Model file for the job. Use its own axes, mm. A direction names the side the tool comes from. Round coordinates to 2 decimals unless told otherwise and drop trailing zeros. Order: outer loops, then holes, each group sorted by start corner. A loop starts at its lowest first (then second) coordinate and runs counter-clockwise, first axis right, second up. Notation, with made-up numbers: (68.5, 23) - (76.5, 23) arc R20 ccw to (76.5, 52) - close; hole circle Ø6 at (1.25, 70). An arc over 180 degrees is marked (long way). Put each result on its own line as item: value. Start each with the question number.
Item 1: Saw through at A-A on y = 23.9. List the corners of the cut face in (x, z).
Item 2: Which spindle directions (+Z, -Z, +X, -X, +Y, -Y) get a long thin tool onto all of the face, cutting with end or side? Do faces 1 (the face through (-20.5, 31, -12)), 2 (the face through (-24, 7.8, -1)), 3 (the face through (24.86, 32.1, -0.57)). Say none if no direction does.
Item 3: Saw through at C-C on x = -24.2. List the corners of the cut face in (y, z).
Item 4: Pin check, flat tips, straight feed: pin 1 Ø2.5 at (x, z) = (26.5, -17) entering from -Y; pin 2 Ø1.3 at (x, z) = (-19.5, -1.5) entering from +Y; pin 3 Ø4.5 at (x, z) = (-10.6, -9) entering from +Y. Stop position of each tip, or through.
Item 5: Probe probe 1 along X at (y, z) = (32, -19.1); probe 2 along Z at (x, y) = (-24, 31); probe 3 along Z at (x, y) = (10, 1). List the from-to ranges inside material, lowest first.
Item 6: Saw through at B-B on x = 4. List the corners of the cut face in (y, z).
Item 7: Mould opens along Z. For faces 4 (the face through (3.247, 1.115, -14.433)), 5 (the face through (29.1, 31, -8)), 6 (the face through (0.3, 0.6, -0.57)) say: pulls with the +Z half, pulls with the -Z half, needs draft (parallel to the pull), parting line crosses it, or undercut.
Item 8: Saw through at D-D on z = -15.8. State how many separate pieces and enclosed holes the cut face has, plus the area to 3 significant figures.
```python
from build123d import *

# Parameters (mm, degrees)
BOSS_EXTRUDE1_DEPTH = 29.1
CUT_EXTRUDE1_DEPTH  = 9.5
SKETCH3_W           = 8.6
SKETCH3_H           = 25.5
CUT_EXTRUDE2_DEPTH  = 4
SKETCH4_W           = 7.8
SKETCH4_H           = 27.6
CUT_EXTRUDE3_DEPTH  = 7.8
SKETCH5_R           = 1.9
CUT_EXTRUDE4_DEPTH  = 2.3
SKETCH6_R           = 1.9
CUT_EXTRUDE5_DEPTH  = 2.1
FILLET_2MM_R        = 2
FILLET2_R           = 0.5
SKETCH7_R           = 1.4
CUT_EXTRUDE6_DEPTH  = 2.2


with BuildPart() as part:
    # Sketch1 → Boss-Extrude1 (new body, symmetric)
    with BuildSketch(Plane(origin=(0, 0, 0), x_dir=(0, 0, -1), z_dir=(1, 0, 0))):
        Polygon((0, 0), (0, 36.7), (25.5, 36.7), (25.5, 30.4), (2.1, 30.4), (2.1, 2.2), (27.6, 2.2), (27.6, 0), align=None)
    extrude(amount=BOSS_EXTRUDE1_DEPTH, both=True)

    # Sketch2 → Cut-Extrude1 (cut)
    with BuildSketch(Plane(origin=(0, 36.7, 0), x_dir=(1, 0, 0), z_dir=(0, 1, 0))):
        Polygon((-18.35, 2.1), (18.35, 2.1), (18.35, 0), (20.5, 0), (20.5, 25.5), (-20.5, 25.5), (-20.5, 0), (-18.35, 0), align=None)
    extrude(amount=-CUT_EXTRUDE1_DEPTH, mode=Mode.SUBTRACT)

    # Sketch3 → Cut-Extrude2 (cut)
    with BuildSketch(Plane(origin=(0, 36.7, 0), x_dir=(1, 0, 0), z_dir=(0, 1, 0))):
        with Locations((24.8, 12.75)):
            Rectangle(SKETCH3_W, SKETCH3_H)
        with Locations((-24.8, 12.75)):
            Rectangle(SKETCH3_W, SKETCH3_H)
    extrude(amount=-CUT_EXTRUDE2_DEPTH, mode=Mode.SUBTRACT)

    # Sketch4 → Cut-Extrude3 (cut)
    with BuildSketch(Plane.XZ):
        with Locations((-25.2, -13.8)):
            Rectangle(SKETCH4_W, SKETCH4_H)
        with Locations((25.2, -13.8)):
            Rectangle(SKETCH4_W, SKETCH4_H)
    extrude(amount=-CUT_EXTRUDE3_DEPTH, mode=Mode.SUBTRACT)

    # Sketch5 → Cut-Extrude4 (cut)
    with BuildSketch(Plane(origin=(0, 32.7, 0), x_dir=(1, 0, 0), z_dir=(0, 1, 0))):
        with Locations((-24.25, 19.1)):
            Circle(SKETCH5_R)
        with Locations((-24.25, 9.1)):
            Circle(SKETCH5_R)
        with Locations((24.25, 9.1)):
            Circle(SKETCH5_R)
        with Locations((24.25, 19.1)):
            Circle(SKETCH5_R)
    extrude(amount=-CUT_EXTRUDE4_DEPTH, mode=Mode.SUBTRACT)

    # Sketch6 → Cut-Extrude5 (cut)
    with BuildSketch(Plane.XY):
        with Locations((24.2, 23.9)):
            Circle(SKETCH6_R)
        with Locations((24.2, 13.9)):
            Circle(SKETCH6_R)
        with Locations((-24.2, 13.9)):
            Circle(SKETCH6_R)
        with Locations((-24.2, 23.9)):
            Circle(SKETCH6_R)
    extrude(amount=-CUT_EXTRUDE5_DEPTH, mode=Mode.SUBTRACT)

    # Fillet 2mm
    fillet_2mm_edges = [part.edges().sort_by_distance(p)[0] for p in [
        (0, 0, 0),
        (-21.3, 1.1, -27.6),
        (-29.1, 7.8, -1.05),
        (29.1, 7.8, -1.05),
        (21.3, 1.1, -27.6),
        (29.1, 31.55, -25.5),
        (-20.5, 31.55, -25.5),
        (20.5, 31.55, -25.5),
        (-18.35, 36.7, -1.05),
        (18.35, 36.7, -1.05),
        (24.8, 32.7, 0),
        (-24.8, 32.7, 0),
        (-29.1, 31.55, -25.5),
    ]]
    fillet(fillet_2mm_edges, radius=FILLET_2MM_R)

    # Fillet2
    fillet2_edges = [part.edges().sort_by_distance(p)[0] for p in [
        (0, 2.2, -2.1),
        (-21.3, 7.8, -1.05),
        (21.3, 7.8, -1.05),
        (24.8, 30.4, -2.1),
        (-24.8, 30.4, -2.1),
        (20.5, 27.2, -1.05),
        (-20.5, 27.2, -1.05),
        (18.35, 27.2, -1.05),
        (-18.35, 27.2, -1.05),
    ]]
    fillet(fillet2_edges, radius=FILLET2_R)

    # Sketch7 → Cut-Extrude6 (cut)
    with BuildSketch(Plane(origin=(0, 2.2, 0), x_dir=(1, 0, 0), z_dir=(0, 1, 0))):
        with Locations((10.6, 22.6)):
            Circle(SKETCH7_R)
        with Locations((10.6, 9)):
            Circle(SKETCH7_R)
        with Locations((10.6, 15.8)):
            Circle(SKETCH7_R)
        with Locations((3.55, 15.8)):
            Circle(SKETCH7_R)
        with Locations((17.65, 15.8)):
            Circle(SKETCH7_R)
        with Locations((-17.65, 15.8)):
            Circle(SKETCH7_R)
        with Locations((-3.55, 15.8)):
            Circle(SKETCH7_R)
        with Locations((-10.6, 15.8)):
            Circle(SKETCH7_R)
        with Locations((-10.6, 9)):
            Circle(SKETCH7_R)
        with Locations((-10.6, 22.6)):
            Circle(SKETCH7_R)
    extrude(amount=-CUT_EXTRUDE6_DEPTH, mode=Mode.SUBTRACT)


solid = part.part
```
Results found:
1. outline: (-29.1, -2.1) - (-26.1, -2.1) - (-26.1, 0) - (-29.1, 0) - close; (-22.3, -2.1) - (22.3, -2.1) - (22.3, 0) - (-22.3, 0) - close; (26.1, -2.1) - (29.1, -2.1) - (29.1, 0) - (26.1, 0) - close
2. face 1: +Z, -Z, +Y
2. face 2: +Z, -Z, -X, -Y
2. face 3: +Z, +X, +Y
3. outline: (7.8, -2.1) - (12, -2.1) - (12, 0) - (7.8, 0) - close; (15.8, -2.1) - (22, -2.1) - (22, 0) - (15.8, 0) - close; (25.8, -2.1) - (29.9, -2.1) arc R0.5 cw to (30.4, -2.6) - (30.4, -7.2) - (32.7, -7.2) - (32.7, -2) arc R2 ccw to (30.7, 0) - (25.8, 0) - close; (30.4, -25.5) - (32.7, -25.5) - (32.7, -21) - (30.4, -21) - close; (30.4, -17.2) - (32.7, -17.2) - (32.7, -11) - (30.4, -11) - close
4. pin 1: stops at y = 30.4
4. pin 2: stops at y = 27.22
4. pin 3: stops at y = 2.2
5. probe 1: x = -29.1 to -26.15, -22.35 to -20.5, 20.5 to 22.35, 26.15 to 29.1
5. probe 2: z = -25.5 to -20.98, -17.22 to -10.98, -7.22 to -0.02
5. probe 3: z = -27.6 to -23.86, -21.34 to -17.06, -14.54 to -10.26, -7.74 to -0.27
6. outline: (0, -27.6) - (2.2, -27.6) - (2.2, -17.13) - (0, -17.13) - close; (0, -14.47) - (2.2, -14.47) - (2.2, -2.6) arc R0.5 cw to (2.7, -2.1) - (36.7, -2.1) - (36.7, 0) - (2, 0) arc R2 ccw to (0, -2) - close
7. face 4: undercut
7. face 5: needs draft
7. face 6: pulls with the +Z half
8. separate pieces: 9
8. enclosed holes: 0
8. area: 96.3 mm²
